Autodesk Inventor part; units mm, degrees
ref_plane "РабПлоскость1" through (0, -0.4556, -12.0524) normal (0.711, -0.0009, 0.7032) x (0, 1, 0.0013)
ref_plane "YZ Plane" through (0, 0, 0) normal (1, 0, 0) x (0, 1, 0)
ref_plane "XZ Plane" through (0, 0, 0) normal (0, 1, 0) x (-1, 0, 0)
sketch "Эскиз1" plane through (0, 0, 0) normal (0, 1, 0) x (-1, 0, 0)
  circle A0 centre (0, 0) radius 5
  circle A1 centre (0, 0) radius 2.6
  circle A2 centre (0, 0) radius 11
  circle A3 centre (8, 0) radius 1.55
  circle A4 centre (-8, 0) radius 1.55
  circle A5 centre (0, 8) radius 1.55
  circle A6 centre (0, -8) radius 1.55
  dimension "d0" = 5.2
  dimension "d1" = 10
  dimension "d2" = 22
  dimension "d3" = 3.1
  dimension "d4" = 3.1
  dimension "d5" = 16
  dimension "d6" = 8
  dimension "d7" = 3.1
  dimension "d8" = 3.1
  dimension "d9" = 8
  dimension "d10" = 8
  dimension "d11" = 16
extrude "Выдавливание1" add sketch "Эскиз1" along normal blind 2 contours A2
extrude "Выдавливание2" add sketch "Эскиз1" along normal blind 12 contours A0
sketch "Эскиз2" plane through (0, 0, 0) normal (1, 0, 0) x (0, 1, 0)
  point P0 (0, 0)
  point P1 (-0.4556, -12.0524)
  point P2 (8.9773, -12.0404)
sketch "Эскиз3" plane through (0, 0, 0) normal (0, 0, 1) x (1, 0, 0)
  point P0 (0, 0)
  point P1 (-11.9191, -0.1213)
  point P2 (-11.9191, 9.5232)
ref_plane "РабПлоскость1" through (0, -0.4556, -12.0524) normal (0.711, -0.0009, 0.7032) x (0, 1, 0.0013)
sketch "Эскиз4" plane through (0, -0.4556, -12.0524) normal (0.711, -0.0009, 0.7032) x (0, 1, 0.0013)
  circle A0 centre (6.1565, 8.569) radius 1.5
  point P0 (0.4709, 8.569)
  dimension "d16" = 3
extrude "Выдавливание3" cut sketch "Эскиз4" along normal up to surface
properties part number "Муфта"
Verification items for the finished model (mm, model axes). Coordinates: 2 decimals unless noted, no trailing zeros. Loops run counter-clockwise (first coordinate to the right, second up) from the corner with the lowest first, then second, coordinate; pieces in that order, holes last. Notation, with made-up numbers: (13, 35) -> (59, 35) arc R24 ccw to (59, 46) -> close; hole circle Ø11 at (73.25, -3.75). An arc over 180 degrees is marked (long way). Answer as a JSON object with one key per item and string values. Group by question number.
Item 1: Sectioned sample at B-B on y = 1.5. Record the boundary of the cut face in (x, z), plus the area to 3 significant figures.
Item 2: Sectioned sample at D-D on z = -8. Record the boundary of the cut face in (x, y), plus the area to 3 significant figures.
Item 3: Depth check by flat-ended pin: pin 1 (4 mm diameter, centred on x = -4.5, y = 2.5, fed in from -Z); pin 2 (2 mm diameter, centred on y = 8, z = -2.5, fed in from -X); pin 3 (3 mm diameter, centred on x = -8, z = 0, fed in from +Y); pin 4 (3.5 mm diameter, centred on x = 0, z = 8, fed in from +Y). Enter the tip coordinate at first touch or a pass-through.
Item 4: Mould release check, pull along Z, two halves, no side actions. Record for faces 1 (the cylindrical face through (6.522, 0.986, -0.466)), 2 (the cylindrical face through (1.08, 6.93, 4.88)), 3 (the flat face through (-2, 2, -5)): +Z half, -Z half, draft (parallel to the pull), parting line (faces both ways), or undercut.
Item 5: Scan lines: probe 1 along Z at (x, y) = (0, 1.3); probe 2 along Z at (x, y) = (0, 7.25); probe 3 along Y at (x, z) = (2.5, -8). Record each from-to range of solid material in increasing order.
Item 6: Sectioned sample at C-C on x = 0.75. Record the boundary of the cut face in (y, z), plus the area to 3 significant figures.
Item 7: Sectioned sample at A-A on z = 0. Record the boundary of the cut face in (x, y).
Evaluation:
{
 "1": {"outline": "circle Ø22 at (0, 0); hole circle Ø3.1 at (-8, 0); hole circle Ø5.2 at (0, 0); hole circle Ø3.1 at (0, -8); hole circle Ø3.1 at (0, 8); hole circle Ø3.1 at (8, 0)", "area": "329 mm²"},
 "2": {"outline": "(-7.55, 0) -> (-1.55, 0) -> (-1.55, 2) -> (-7.55, 2) -> close; (1.55, 0) -> (7.55, 0) -> (7.55, 2) -> (1.55, 2) -> close", "area": "24.0 mm²"},
 "3": {"pin 1": "stops at z = -10.7", "pin 2": "stops at x = -4.77", "pin 3": "passes through", "pin 4": "stops at y = 2"},
 "4": {"face 1": "undercut", "face 2": "parting line", "face 3": "draft"},
 "5": {"probe 1": "z = -11 to -9.55, -6.45 to -2.6, 2.6 to 6.45, 9.55 to 11", "probe 2": "z = -5 to -2.6, 2.6 to 5", "probe 3": "y = 0 to 2"},
 "6": {"outline": "(0, -10.97) -> (2, -10.97) -> (2, -9.36) -> (0, -9.36) -> close; (0, -6.64) -> (2, -6.64) -> (2, -4.94) -> (12, -4.94) -> (12, -2.49) -> (0, -2.49) -> close; (0, 2.49) -> (12, 2.49) -> (12, 4.94) -> (2, 4.94) -> (2, 6.64) -> (0, 6.64) -> close; (0, 9.36) -> (2, 9.36) -> (2, 10.97) -> (0, 10.97) -> close", "area": "72.2 mm²"},
 "7": {"outline": "(-11, 0) -> (-9.55, 0) -> (-9.55, 2) -> (-11, 2) -> close; (-6.45, 0) -> (-2.6, 0) -> (-2.6, 12) -> (-5, 12) -> (-5, 2) -> (-6.45, 2) -> close; (2.6, 0) -> (6.45, 0) -> (6.45, 2) -> (5, 2) -> (5, 12) -> (2.6, 12) -> close; (9.55, 0) -> (11, 0) -> (11, 2) -> (9.55, 2) -> close"}
}
